Part model, mm, in its own coordinate system. Face numbers are marked on the shaded views. A direction names the side the tool comes from. Give positions to 0.01 mm unless a question says otherwise; leave off trailing zeros. Loops run counter-clockwise (first coordinate to the right, second up) from the corner with the lowest first, then second, coordinate; pieces in that order, holes last. Notation, with made-up numbers: (-3.5, 10.25) -> (25.5, 10.25) arc R9 cw to (25.5, 18.25) -> close; hole circle Ø2 at (-4.75, 6.25). An arc over 180 degrees is marked (long way). Write item = value, one per line.
from build123d import *

# Parameters (mm, degrees)
SKETCH_1_R          = 20
EXTRUDE_1_DEPTH     = 100
SKETCH_2_R          = 30
EXTRUDE_2_DEPTH     = 8
SKETCH_3_R          = 30
EXTRUDE_3_DEPTH     = 8
SKETCH_4_R          = 15
EXTRUDE_4_DEPTH     = 60
SKETCH_5_R          = 15
CUT_EXTRUDE_1_DEPTH = 121.415945838
SKETCH_7_R          = 11
CUT_EXTRUDE_3_DEPTH = 60
SKETCH_8_R          = 3
CUT_EXTRUDE_4_DEPTH = 8
CUT_EXTRUDE_START   = -8
SKETCH_9_R          = 3
CUT_EXTRUDE_5_DEPTH = 8


with BuildPart() as part:
    # 草图1 → 凸台-拉伸1 (new body)
    with BuildSketch(Plane(origin=(-50, 0, 0), x_dir=(0, 0, -1), z_dir=(1, 0, 0))):
        Circle(SKETCH_1_R)
    extrude(amount=EXTRUDE_1_DEPTH)

    # 草图2 → 凸台-拉伸2 (add)
    with BuildSketch(Plane(origin=(-50, 0, 0), x_dir=(0, 0, -1), z_dir=(1, 0, 0))):
        Circle(SKETCH_2_R)
    extrude(amount=EXTRUDE_2_DEPTH)

    # 草图3 → 凸台-拉伸3 (add)
    with BuildSketch(Plane(origin=(42, 0, 0), x_dir=(0, 0, -1), z_dir=(1, 0, 0))):
        Circle(SKETCH_3_R)
    extrude(amount=EXTRUDE_3_DEPTH)

    # 草图4 → 凸台-拉伸4 (add)
    with BuildSketch(Plane(origin=(0, 0, 0), x_dir=(1, 0, 0), z_dir=(0, 1, 0))):
        with Locations(Location((0, 0, 0), (0, 0, 90))):
            Circle(SKETCH_4_R)
    extrude(amount=EXTRUDE_4_DEPTH)

    # 草图5 → 切除-拉伸1 (cut, through all)
    with BuildSketch(Plane(origin=(-50, 0, 0), x_dir=(0, 0, -1), z_dir=(1, 0, 0))):
        Circle(SKETCH_5_R)
    extrude(amount=CUT_EXTRUDE_1_DEPTH, mode=Mode.SUBTRACT)

    # 草图7 → 切除-拉伸3 (cut)
    with BuildSketch(Plane(origin=(0, 60, 0), x_dir=(1, 0, 0), z_dir=(0, 1, 0))):
        with Locations(Location((0, 0, 0), (0, 0, 270))):
            Circle(SKETCH_7_R)
    extrude(amount=-CUT_EXTRUDE_3_DEPTH, mode=Mode.SUBTRACT)

    # 草图8 → 切除-拉伸4 (cut)
    with BuildSketch(Plane(origin=(-50, 0, 0), x_dir=(0, 0, -1), z_dir=(1, 0, 0))):
        with Locations((-16.970563, 16.970563)):
            Circle(SKETCH_8_R)
        with Locations((16.970563, 16.970563)):
            Circle(SKETCH_8_R)
        with Locations((16.970563, -16.970563)):
            Circle(SKETCH_8_R)
        with Locations((-16.970563, -16.970563)):
            Circle(SKETCH_8_R)
    extrude(amount=CUT_EXTRUDE_4_DEPTH, mode=Mode.SUBTRACT)

    # 草图9 → 切除-拉伸5 (cut)
    with BuildSketch(Plane(origin=(50, 0, 0), x_dir=(0, 0, -1), z_dir=(1, 0, 0)).offset(CUT_EXTRUDE_START)):
        with Locations((-16.970563, 16.970563)):
            Circle(SKETCH_9_R)
        with Locations((16.970563, 16.970563)):
            Circle(SKETCH_9_R)
        with Locations((16.970563, -16.970563)):
            Circle(SKETCH_9_R)
        with Locations((-16.970563, -16.970563)):
            Circle(SKETCH_9_R)
    extrude(amount=CUT_EXTRUDE_5_DEPTH, mode=Mode.SUBTRACT)


solid = part.part
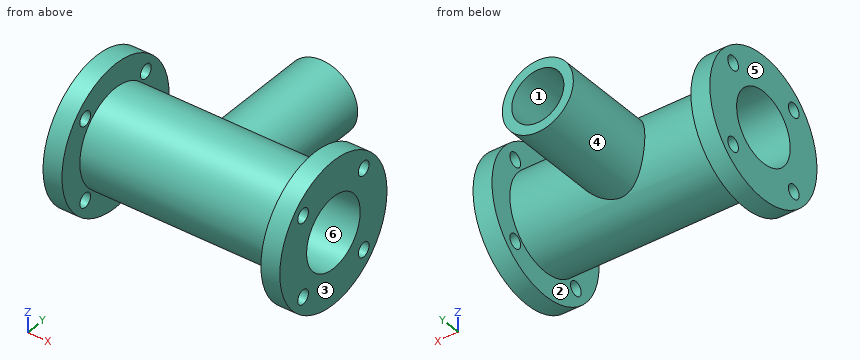
1) Drop flat-ended pins along their axis: P1, Ø2, axis at x = 2, y = 35, coming from the +Z side; P2, Ø12, axis at x = 29.5, y = -12.5, coming from the +Z side; P3, Ø12, axis at x = -19.5, z = -13, coming from the +Y side (3 decimals); P4, Ø9.5, axis at y = 16.97, z = -16.97, coming from the +X side. Give the stop position or say it passes through.
Resolved:
P1 = 14.97
P2 = 18.91
P3 = 18.735
P4 = 50
2) Slice it at D-D, the plane z = -18.5. List the corners of the cut face in (x, y).
Resolved:
outline = (-50, -23.62) -> (-42, -23.62) -> (-42, -19.55) -> (-50, -19.55) -> close; (-50, -14.39) -> (-42, -14.39) -> (-42, -7.6) -> (42, -7.6) -> (42, -14.39) -> (50, -14.39) -> (50, 14.39) -> (42, 14.39) -> (42, 7.6) -> (-42, 7.6) -> (-42, 14.39) -> (-50, 14.39) -> close; (-50, 19.55) -> (-42, 19.55) -> (-42, 23.62) -> (-50, 23.62) -> close; (42, -23.62) -> (50, -23.62) -> (50, -19.55) -> (42, -19.55) -> close; (42, 19.55) -> (50, 19.55) -> (50, 23.62) -> (42, 23.62) -> close
3) Slice it at B-B, the plane z = 0. List the corners of the cut face in (x, y).
Resolved:
outline = (-50, -30) -> (-42, -30) -> (-42, -20) -> (42, -20) -> (42, -30) -> (50, -30) -> (50, -15) -> (-50, -15) -> close; (-50, 15) -> (-11, 15) -> (-11, 60) -> (-15, 60) -> (-15, 20) -> (-42, 20) -> (-42, 30) -> (-50, 30) -> close; (11, 15) -> (50, 15) -> (50, 30) -> (42, 30) -> (42, 20) -> (15, 20) -> (15, 60) -> (11, 60) -> close
4) Slice it at A-A, the plane y = 0. List the corners of the cut face in (x, z), and give its area (3 significant figures).
Resolved:
outline = (-50, -30) -> (-42, -30) -> (-42, -20) -> (42, -20) -> (42, -30) -> (50, -30) -> (50, -15) -> (-50, -15) -> close; (-50, 15) -> (50, 15) -> (50, 30) -> (42, 30) -> (42, 20) -> (-42, 20) -> (-42, 30) -> (-50, 30) -> close
area = 1,320 mm²
5) Drill centre lines: line 1 along X through (y, z) = (5.5, -20); line 2 along Y through (x, z) = (-30, 8); line 3 along Z through (x, y) = (0.5, 46.5). Where is each one in solid material? Low to high. Write a range as [from, to].
Resolved:
line_1 = [-50, -42], [42, 50]
line_2 = [-18.33, -12.69], [12.69, 18.33]
line_3 = [-14.99, -10.99], [10.99, 14.99]
6) Which spindle directions (+Z, -Z, +X, -X, +Y, -Y) get a long thin tool onto all of the face, cutting with end or side? Do the marked faces 1, 2 and 3. Say none if no direction does.
Resolved:
face_1 = +Y
face_2 = none
face_3 = +Z, -Z, +X, +Y, -Y
7) Slice it at C-C, the plane x = 0. List the corners of the cut face in (y, z).
Resolved:
outline = (10.2, -11) arc R15 cw (long way) to (10.2, 11) -> (60, 11) -> (60, 15) -> (13.23, 15) arc R20 ccw (long way) to (13.23, -15) -> (60, -15) -> (60, -11) -> close
8) Pull direction Z, two halves, no side cores. Call the marked faces 4, 5 and 6: pulls with the +Z half, pulls with the -Z half, needs draft (parallel to the pull), parting line crosses it, or undercut.
Resolved:
face_4 = parting line crosses it
face_5 = needs draft
face_6 = undercut
